from build123d import *

# Parameters (mm, degrees)
SKETCH1_R                = 11.5
BOSS_EXTRUDE1_DEPTH      = 5
SKETCH2_R                = 2.25
CUT_EXTRUDE1_DEPTH       = 18.014699527
CIRPATTERN1_COUNT        = 4
SKETCH3_R                = 4
BOSS_EXTRUDE2_DEPTH      = 10
SKETCH4_R                = 2.25
CUT_EXTRUDE2_DEPTH       = 23.12464689
BOSS_EXTRUDE3_REACH      = 28.448
BOSS_EXTRUDE3_END_RADIUS = 4
SKETCH5_W                = 8
SKETCH5_H                = 7.5
SKETCH6_R                = 2.25
CUT_EXTRUDE3_DEPTH       = 7
CHAMFER1_SIZE            = 1
CHAMFER2_SIZE            = 1


with BuildPart() as part:
    # Sketch1 → Boss-Extrude1 (new body)
    with BuildSketch(Plane.XY):
        Circle(SKETCH1_R)
    extrude(amount=BOSS_EXTRUDE1_DEPTH)

    # Sketch2 → Cut-Extrude1 (cut, through all)
    with BuildSketch(Plane.XY.offset(5)):
        with Locations((0, 7)):
            Circle(SKETCH2_R)
    cut_extrude1 = extrude(amount=-CUT_EXTRUDE1_DEPTH, mode=Mode.SUBTRACT)

    # CirPattern1: Cut-Extrude1 ×4 about axis
    cirpattern1_axis = Axis((0, 0, 0), (0, 0, 1))
    for i in range(1, CIRPATTERN1_COUNT):
        add(cut_extrude1.rotate(cirpattern1_axis, i * 360 / CIRPATTERN1_COUNT), mode=Mode.SUBTRACT)

    # Sketch3 → Boss-Extrude2 (add)
    with BuildSketch(Plane.XY.offset(5)):
        Circle(SKETCH3_R)
    extrude(amount=BOSS_EXTRUDE2_DEPTH)

    # Sketch4 → Cut-Extrude2 (cut, through all)
    with BuildSketch(Plane.XY.offset(15)):
        Circle(SKETCH4_R)
    extrude(amount=-CUT_EXTRUDE2_DEPTH, mode=Mode.SUBTRACT)

    # Boss-Extrude3: up to this cylinder (the profile starts outside it)
    boss_extrude3_end = Plane(origin=(0, 0, 8.75), z_dir=(0, 0, -1)) * Cylinder(BOSS_EXTRUDE3_END_RADIUS, 65.896, mode=Mode.PRIVATE)
    # Sketch5 → Boss-Extrude3 (add, up to the surface)
    with BuildSketch(Plane(origin=(0, 7, 0), x_dir=(1, 0, 0), z_dir=(0, 1, 0)), mode=Mode.PRIVATE) as boss_extrude3_sk1:
        with Locations((0, -8.75)):
            Rectangle(SKETCH5_W, SKETCH5_H)
    boss_extrude3_tool1 = extrude(boss_extrude3_sk1.sketch, amount=-BOSS_EXTRUDE3_REACH, mode=Mode.PRIVATE) - boss_extrude3_end
    add(boss_extrude3_tool1.solids().sort_by_distance((0, 7, 8.75))[0])

    # Sketch6 → Cut-Extrude3 (cut)
    with BuildSketch(Plane(origin=(0, 7, 0), x_dir=(1, 0, 0), z_dir=(0, 1, 0))):
        with Locations(Location((0, -8.75, 0), (0, 0, 270))):
            Circle(SKETCH6_R)
    extrude(amount=-CUT_EXTRUDE3_DEPTH, mode=Mode.SUBTRACT)

    # Chamfer1
    chamfer1_edges = [part.edges().sort_by_distance(p)[0] for p in [
        (0, 7, 6.5),
    ]]
    chamfer(chamfer1_edges, length=CHAMFER1_SIZE)

    # Chamfer2
    chamfer2_edges = [part.edges().sort_by_distance(p)[0] for p in [
        (-7, -2.25, 0),
        (2.25, -7, 0),
        (7, 2.25, 0),
        (-2.25, 7, 0),
    ]]
    chamfer(chamfer2_edges, length=CHAMFER2_SIZE)


solid = part.part
Design review of the part built by this model. Coordinates are the model's own, in mm. A direction names the side the tool comes from. Round coordinates to 2 decimals unless told otherwise and drop trailing zeros. Write each loop counter-clockwise with the first axis right and the second up, starting at its lowest first coordinate (ties: lowest second). Pieces come first, ordered by that corner, then holes. Notation, with made-up numbers: (11.5, 43.5) -> (63.5, 43.5) arc R21 cw to (63.5, 53.5) -> close; hole circle Ø5 at (-32, 74.25). An arc over 180 degrees is marked (long way). One line per question, with ' | ' between items.
(1) Take a section at D-D, the plane y = 1.75. State how many separate pieces and enclosed holes the cut face has, and give its area (3 significant figures).
Result sheet:
separate pieces: 4 | enclosed holes: 0 | area: 114 mm2
(2) Insertion check: P1, Ø5.5, axis at y = 2, z = 7, coming from the -X side; P2, Ø6, axis at x = -1, z = 9, coming from the +Y side; P3, Ø5, axis at x = 7, y = 0, coming from the -Z side. Each pin has a flat end and moves straight along its axis. Give the tip position at first contact, or say it passes through.
Result sheet:
P1: x = -11.5 | P2: y = 7 | P3: z = 0.75
(3) Take a section at B-B, the plane x = -7. State the section outline as (y, z) points.
Result sheet:
outline: (-9.12, 0) -> (-3.25, 0) -> (-2.25, 1) -> (-2.25, 5) -> (-9.12, 5) -> close; (2.25, 1) -> (3.25, 0) -> (9.12, 0) -> (9.12, 5) -> (2.25, 5) -> close
(4) Wall thickness on line 1 (Y direction, x = 0, z = 3.5); line 2 (Z direction, x = 9, y = -6); line 3 (Y direction, x = -0.75, z = 11): over which ranges is each line inside the solid? List them lowest first. Write a range as [from, to].
Result sheet:
line 1: [-11.5, -9.25], [-4.75, -2.25], [2.25, 4.75], [9.25, 11.5] | line 2: [0, 5] | line 3: [-3.93, -2.12], [2.12, 6.12]
(5) Take a section at A-A, the plane z = 3. State the section outline as (x, y) points.
Result sheet:
outline: circle Ø23 at (0, 0); hole circle Ø4.5 at (-7, 0); hole circle Ø4.5 at (0, -7); hole circle Ø4.5 at (0, 0); hole circle Ø4.5 at (0, 7); hole circle Ø4.5 at (7, 0)
(6) Draft analysis for pull direction Z (two halves, no side actions). For faces 1 (the cylindrical face through (2.23, 3.71, 8.46)), 2 (the flat face through (2, -5, 5)), 3 (the flat face through (2.4, 0.2, 0)), state which applies: released by +Z, released by -Z, zero draft, split by the parting line, or undercut.
Result sheet:
face 1: undercut | face 2: released by +Z | face 3: released by -Z
(7) Take a section at C-C, the plane z = 8.75. State the section outline as (x, y) points, and give its area (3 significant figures).
Result sheet:
outline: (-4, 0) arc R4 ccw to (4, 0) -> (4, 7) -> (3.25, 7) -> (2.25, 6) -> (2.25, 0) arc R2.25 cw to (-2.25, 0) -> (-2.25, 6) -> (-3.25, 7) -> (-4, 7) -> close | area: 40.7 mm2
(8) Machinability: for faces 4 (the flat face through (4, 4, 9)), 5 (the flat face through (-1, 7, 12)), 6 (the cylindrical face through (-0.867, -3.905, 11.041)), 7 (the cylindrical face through (1.21, 8.897, 3.028)), 8 (the cylindrical face through (-1.5, 11.4, 2.5)), which of the approach directions +Z, -Z, +X, -X, +Y, -Y give a long, thin tool a straight path to every point of the face, cutting with its end or side? Answer none if there is none.
Result sheet:
face 4: +Z, +X, +Y, -Y | face 5: +Z, +X, -X, +Y | face 6: +Z | face 7: -Z | face 8: +Z, -Z
